Part model, mm, in its own coordinate system. A direction names the side the tool comes from. Give positions to 0.01 mm unless a question says otherwise; leave off trailing zeros. Write each loop counter-clockwise with the first axis right and the second up, starting at its lowest first coordinate (ties: lowest second). Pieces come first, ordered by that corner, then holes. Notation, with made-up numbers: M 64,-7.5 L 121,-7.5 A19 cw 121,20.5 Z; hole C 32,85.5 d4. An arc over 180 degrees is marked long. Write item = value, one per line. Start each with the question number.
Autodesk Fusion 360 part; units mm, degrees
sketch "Sketch1" plane through (0, 0, 0) normal (0, 0, 1) x (1, 0, 0)
  line L0 (0, 0) -> (75, 0)
  line L1 (75, 0) -> (75, 75)
  line L2 (75, 75) -> (0, 75)
  line L3 (0, 75) -> (0, 0)
  circle A0 centre (37.5, 37.5) radius 11.65
  circle A1 centre (10, 65) radius 1.524
  circle A2 centre (65, 65) radius 1.524
  circle A3 centre (10, 10) radius 1.524
  circle A4 centre (65, 10) radius 1.524
  dimension "d1" = 75
  dimension "d2" = 75
  dimension "d3" = 37.5
  dimension "d4" = 37.5
  dimension "d5" = 23.3
  dimension "d6" = 3.048
  dimension "d7" = 10
  dimension "d8" = 10
  dimension "d9" = 10
  dimension "d10" = 10
  dimension "d11" = 10
  dimension "d12" = 10
  dimension "d13" = 10
  dimension "d14" = 10
extrude "Extrude1" add sketch "Sketch1" along normal blind 7.62
fillet "Fillet1" radius 2 4 edges at (75, 0, 3.81) (75, 75, 3.81) (0, 0, 3.81) (0, 75, 3.81)
sketch "Sketch2" plane through (0, 0, 0) normal (0, -1, 0) x (1, 0, 0)
  line L0 (2, 7.62) -> (2, 0)
  line L1 (2, 0) -> (73, 0)
  line L2 (73, 0) -> (73, 7.62)
  line L3 (73, 7.62) -> (2, 7.62)
  circle A0 centre (37.5, 3.81) radius 1.016
  dimension "d19" = 35.5
  dimension "d20" = 2.032
  dimension "d21" = 3.81
hole "Hole1" at (37.5, 0, 3.81) direction (0, 1, 0) diameter 2.032 depth 30 tip angle 118
Q1. Two-plate mould, pull along Y, no slides. Class faces 1 (the face through (66.454, 9.542, 3.757)), 2 (the face through (29, 46, 0)), 3 (the face through (11.4, 65.6, 3.8)), 4 (the face through (74.4, 0.57, 3.86)): +Y half, -Y half, draft (parallel to the pull), parting line (faces both ways), or undercut.
Q2. Slice it at D-D (y = 37.5). Give the cut face in (x, z), and give its area (3 significant figures).
Q3. Probe line 1 along Y through (x, z) = (10, 3.5); line 2 along Y through (x, z) = (37.5, 2.5). List the from-to ranges inside material, lowest first.
Q4. Slice it at A-A (y = 10). Give the cut face in (x, z), and give its area (3 significant figures).
Q5. Slice it at B-B (y = 65). Give the cut face in (x, z), and give its area (3 significant figures).
Q6. Tool access for faces 5 (the face through (38, 75, 4)), 6 (the face through (36.493, 13.128, 3.942)): list every direction of +Z, -Z, +X, -X, +Y, -Y with a clear straight run to the whole face (end or side of a thin tool).
Working result:
q1.face_1 = undercut
q1.face_2 = draft
q1.face_3 = undercut
q1.face_4 = -Y half
q2.outline = M 0,0 L 25.85,0 L 25.85,7.62 L 0,7.62 Z; M 49.15,0 L 75,0 L 75,7.62 L 49.15,7.62 Z
q2.area = 394 mm2
q3.line_1 = 0 to 8.48, 11.52 to 63.48, 66.52 to 75
q3.line_2 = 0 to 25.85, 49.15 to 75
q4.outline = M 0,0 L 8.48,0 L 8.48,7.62 L 0,7.62 Z; M 11.52,0 L 63.48,0 L 63.48,7.62 L 11.52,7.62 Z; M 66.52,0 L 75,0 L 75,7.62 L 66.52,7.62 Z; hole C 37.5,3.81 d2.03
q4.area = 522 mm2
q5.outline = M 0,0 L 8.48,0 L 8.48,7.62 L 0,7.62 Z; M 11.52,0 L 63.48,0 L 63.48,7.62 L 11.52,7.62 Z; M 66.52,0 L 75,0 L 75,7.62 L 66.52,7.62 Z
q5.area = 525 mm2
q6.face_5 = +Z, -Z, +X, -X, +Y
q6.face_6 = -Y
